```python
from build123d import *

# Parameters (mm, degrees)
BASE_FLANGE1_DEPTH      = 0.7
EDGE_FLANGE1_DEPTH      = 13.370958639
EDGE_FLANGE1_BEND_DEPTH = 15.064251929


# Sheet-metal steps are written as plain solids
with BuildPart() as part:
    # Sketch1 → Base-Flange1 (new body)
    with BuildSketch(Plane(origin=(0, 0, 0), x_dir=(0, 0, -1), z_dir=(1, 0, 0))):
        Polygon((0, 0), (-13.370958639, 0), (33.191160263, -52.458728532), (33.191160263, -37.394476603), align=None)
    extrude(amount=-BASE_FLANGE1_DEPTH)

    # Edge-Flange1 section (across the edge) → Edge-Flange1 (add)
    with BuildSketch(Plane(origin=(0, 0.7366, 0), x_dir=(0, -1, 0), z_dir=(0, 0, 1))):
        with BuildLine():
            Line((-0.7, 0.7366), (-0.7, 15))
            Line((-0.7, 15), (0, 15))
            Line((0, 15), (0, 0.7366))
            ThreePointArc((0, 0.7366), (0.215745145, 0.215745145), (0.7366, 0))
            Line((0.7366, 0), (0.7366, -0.7))
            ThreePointArc((0.7366, -0.7), (-0.279229602, -0.279229602), (-0.7, 0.7366))
        make_face()
    extrude(amount=EDGE_FLANGE1_DEPTH)

    # Edge-Flange1 section 2 (across the edge) → Edge-Flange1 bend (add)
    with BuildSketch(Plane(origin=(0, -52.458728532, -33.927760263), x_dir=(0, 0, 1), z_dir=(0, 1, 0))):
        with BuildLine():
            Line((-0.7, 0.7366), (-0.7, 15))
            Line((-0.7, 15), (0, 15))
            Line((0, 15), (0, 0.7366))
            ThreePointArc((0, 0.7366), (0.215745145, 0.215745145), (0.7366, 0))
            Line((0.7366, 0), (0.7366, -0.7))
            ThreePointArc((0.7366, -0.7), (-0.279229602, -0.279229602), (-0.7, 0.7366))
        make_face()
    extrude(amount=EDGE_FLANGE1_BEND_DEPTH)


solid = part.part
```
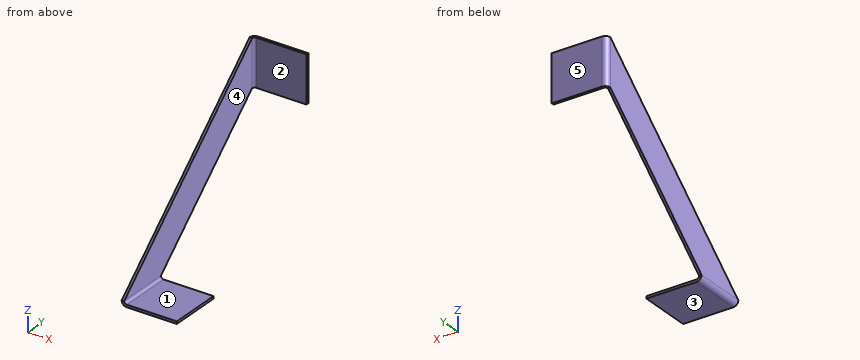
Could you check a few things on this model? Use its own coordinates, in mm. Face numbers are marked on the shaded views. A direction names the side the tool comes from. Round coordinates to 2 decimals unless told otherwise and drop trailing zeros. Write each loop counter-clockwise with the first axis right and the second up, starting at its lowest first coordinate (ties: lowest second). Pieces come first, ordered by that corner, then holes.
(1) Suppose I cut it at A-A on x = 4.75. Write out the boundary of the cut face in (y, z), and give its area (3 significant figures).
Findings below:
outline: (-52.46, -34.63) - (-37.39, -34.63) - (-37.39, -33.93) - (-52.46, -33.93) - close; (0.74, 0) - (1.44, 0) - (1.44, 13.37) - (0.74, 13.37) - close
area: 19.9 mm2
(2) Suppose I cut it at B-B on z = 6. Write out the boundary of the cut face in (x, y).
Findings below:
outline: (-0.7, -8.3) - (0, -8.3) - (0, 0) arc R0.74 cw to (0.74, 0.74) - (15, 0.74) - (15, 1.44) - (0.74, 1.44) arc R1.44 ccw to (-0.7, 0) - close
(3) Suppose I cut it at C-C on y = -17. Write out the boundary of the cut face in (x, z), and give its area (3 significant figures).
Findings below:
outline: (-0.7, -15.09) - (0, -15.09) - (0, -1.72) - (-0.7, -1.72) - close
area: 9.36 mm2
(4) If I drill on probe 1 along X at (y, z) = (-10, -6); probe 2 along Z at (x, y) = (1.5, -43); probe 3 along Y at (x, z) = (6.75, 2), over which ranges is the centre line in solid material (lowest first)?
Findings below:
probe 1: x = -0.7 to 0
probe 2: z = -34.63 to -33.93
probe 3: y = 0.74 to 1.44
(5) For pin 1 (1.1 mm diameter, centred on x = 7, z = -33.5, fed in from +Y); pin 2 (1.6 mm diameter, centred on x = 5, y = 1, fed in from -Z); pin 3 (7 mm diameter, centred on x = 8, y = -47, fed in from +Z); pin 4 (2 mm diameter, centred on y = -18.5, z = -19, fed in from -X), each with a flat end and sliding along its axis, tell me the tip position at first contact or that it passes through.
Findings below:
pin 1: stops at y = -37.39
pin 2: stops at z = 0
pin 3: stops at z = -33.93
pin 4: passes through
(6) Suppose I cut it at D-D on z = -24. Write out the boundary of the cut face in (x, y).
Findings below:
outline: (-0.7, -42.1) - (0, -42.1) - (0, -27.04) - (-0.7, -27.04) - close
(7) Which directions (+Z, -Z, +X, -X, +Y, -Y) give clear straight access to the entire face, cutting with the end or side of a thin tool? Please do the marked faces 1, 2, 3, 4 and 5.
Findings below:
face 1: +Z, +X, +Y, -Y
face 2: +Z, -Z, +X, -Y
face 3: -Z, +X, -X, +Y, -Y
face 4: +Z, +X, -Y
face 5: +Z, -Z, +X, -X, +Y
